The model under review builds one solid part; all positions refer to its coordinate system, in mm. A direction names the side the tool comes from. Give positions to 0.01 mm unless a question says otherwise; leave off trailing zeros. Order: outer loops, then holes, each group sorted by start corner. A loop starts at its lowest first (then second) coordinate and runs counter-clockwise, first axis right, second up.
```python
from build123d import *

# Parameters (mm, degrees)
SKETCH1_R           = 12
SKETCH1_R_2         = 10.5
BOSS_EXTRUDE1_DEPTH = 3
CUT_EXTRUDE1_DEPTH  = 1
CUT_EXTRUDE2_DEPTH  = 3
CUT_EXTRUDE3_DEPTH  = 1


with BuildPart() as part:
    # Sketch1 → Boss-Extrude1 (new body)
    with BuildSketch(Plane(origin=(0, 0, 0), x_dir=(1, 0, 0), z_dir=(0, 1, 0))):
        Circle(SKETCH1_R)
        Circle(SKETCH1_R_2, mode=Mode.SUBTRACT)
    extrude(amount=-BOSS_EXTRUDE1_DEPTH)

    # Sketch6 → Cut-Extrude1 (cut)
    with BuildSketch(Plane(origin=(0, 0, 0), x_dir=(1, 0, 0), z_dir=(0, 1, 0))):
        with BuildLine():
            Line((10.246950766, 4), (11.313708499, 4))
            ThreePointArc((11.313708499, 4), (12, 0), (11.313708499, -4))
            Line((11.313708499, -4), (10.246950766, -4))
            ThreePointArc((10.246950766, -4), (11, 0), (10.246950766, 4))
        make_face()
        with BuildLine():
            Line((-4, 10.246950766), (-4, 11.313708499))
            ThreePointArc((-4, 11.313708499), (0, 12), (4, 11.313708499))
            Line((4, 11.313708499), (4, 10.246950766))
            ThreePointArc((4, 10.246950766), (0, 11), (-4, 10.246950766))
        make_face()
        with BuildLine():
            Line((4, -10.246950766), (4, -11.313708499))
            ThreePointArc((4, -11.313708499), (0, -12), (-4, -11.313708499))
            Line((-4, -11.313708499), (-4, -10.246950766))
            ThreePointArc((-4, -10.246950766), (0, -11), (4, -10.246950766))
        make_face()
        with BuildLine():
            Line((-10.246950766, -4), (-11.313708499, -4))
            ThreePointArc((-11.313708499, -4), (-12, 0), (-11.313708499, 4))
            Line((-11.313708499, 4), (-10.246950766, 4))
            ThreePointArc((-10.246950766, 4), (-11, 0), (-10.246950766, -4))
        make_face()
    extrude(amount=-CUT_EXTRUDE1_DEPTH, mode=Mode.SUBTRACT)

    # Sketch7 → Cut-Extrude2 (cut, through all)
    with BuildSketch(Plane(origin=(0, -1, 0), x_dir=(1, 0, 0), z_dir=(0, 1, 0))):
        with BuildLine():
            Line((-2, 10.816653826), (-2, 11.832159566))
            ThreePointArc((-2, 11.832159566), (0, 12), (2, 11.832159566))
            Line((2, 11.832159566), (2, 10.816653826))
            ThreePointArc((2, 10.816653826), (0, 11), (-2, 10.816653826))
        make_face()
        with BuildLine():
            Line((10.816653826, -2), (11.832159566, -2))
            ThreePointArc((11.832159566, -2), (12, 0), (11.832159566, 2))
            Line((11.832159566, 2), (10.816653826, 2))
            ThreePointArc((10.816653826, 2), (11, 0), (10.816653826, -2))
        make_face()
        with BuildLine():
            Line((-2, -10.816653826), (-2, -11.832159566))
            ThreePointArc((-2, -11.832159566), (0, -12), (2, -11.832159566))
            Line((2, -11.832159566), (2, -10.816653826))
            ThreePointArc((2, -10.816653826), (0, -11), (-2, -10.816653826))
        make_face()
        with BuildLine():
            Line((-10.816653826, 2), (-11.832159566, 2))
            ThreePointArc((-11.832159566, 2), (-12, 0), (-11.832159566, -2))
            Line((-11.832159566, -2), (-10.816653826, -2))
            ThreePointArc((-10.816653826, -2), (-11, 0), (-10.816653826, 2))
        make_face()
    extrude(amount=-CUT_EXTRUDE2_DEPTH, mode=Mode.SUBTRACT)

    # Sketch8 → Cut-Extrude3 (cut)
    with BuildSketch(Plane.XZ.offset(3)):
        with BuildLine():
            Line((-5, -9.233092656), (-5, -10.908712115))
            ThreePointArc((-5, -10.908712115), (-5.764655514, -10.52467324), (-6.5, -10.087120501))
            Line((-6.5, -10.087120501), (-6.5, -8.246211251))
            ThreePointArc((-6.5, -8.246211251), (-5.77113366, -8.771773838), (-5, -9.233092656))
        make_face()
        with BuildLine():
            Line((5, -9.233092656), (5, -10.908712115))
            ThreePointArc((5, -10.908712115), (5.764655514, -10.52467324), (6.5, -10.087120501))
            Line((6.5, -10.087120501), (6.5, -8.246211251))
            ThreePointArc((6.5, -8.246211251), (5.77113366, -8.771773838), (5, -9.233092656))
        make_face()
    extrude(amount=-CUT_EXTRUDE3_DEPTH, mode=Mode.SUBTRACT)


solid = part.part
```
1. Take a section at D-D (x = 3.25). Write out the cut boundary in (y, z).
2. For faces 4 (the flat face through (-4, -0.5, 10.8)), 5 (the flat face through (-6.5, -2.5, -9.2)), 6 (the flat face through (2, -2, 11)), list the 3-axis set-ups (+Z, -Z, +X, -X, +Y, -Y) from which the entire face can be reached by the end or side of a thin tool; tool diameter is ignored.
3. Take a section at C-C (y = -0.55). Write out the cut boundary in (x, z).
4. Insertion check: pin 1 (1.1 mm diameter, centred on y = -0.5, z = -10.5, fed in from +X); pin 2 (0.5 mm diameter, centred on x = 11, z = 3.5, fed in from +Y); pin 3 (0.5 mm diameter, centred on y = -1.5, z = 11, fed in from -X); pin 4 (6 mm diameter, centred on x = -4.5, z = -3, fed in from +Y). Each pin has a flat end and moves straight along its axis. Give the tip position at first contact, or say it passes through.
5. Take a section at B-B (x = 0). Write out the cut boundary in (y, z), and give its area (3 significant figures).
6. To check wall thickness, follow line 1 (Z direction, x = 0, y = -1.7); line 2 (X direction, y = -0.4, z = 6.5). State the ranges of each line that lie inside material, in increasing order.
7. Draft analysis for pull direction X (two halves, no side actions). For faces 1 (the cylindrical face through (-8.41, -1.48, -8.56)), 2 (the flat face through (11, -2, 2)), 3 (the flat face through (4, -0.5, 10.8)), state which applies: pulls with the +X half, pulls with the -X half, needs draft (parallel to the pull), parting line crosses it, or undercut.
8. Take a section at A-A (z = 0). Write out the cut boundary in (x, y), and give its area (3 significant figures).
Answer:
1. outline: (-3, -11.55) - (-1, -11.55) - (-1, -10.51) - (0, -10.51) - (0, -9.98) - (-3, -9.98) - close; (-3, 9.98) - (0, 9.98) - (0, 10.51) - (-1, 10.51) - (-1, 11.55) - (-3, 11.55) - close
2. face 4: +Z, +Y
2. face 5: -Z, -Y
2. face 6: +Z, +Y, -Y
3. outline: (-11.31, -4) arc R12 ccw to (-4, -11.31) - (-4, -10.25) arc R11 ccw to (4, -10.25) - (4, -11.31) arc R12 ccw to (11.31, -4) - (10.25, -4) arc R11 ccw to (10.25, 4) - (11.31, 4) arc R12 ccw to (4, 11.31) - (4, 10.25) arc R11 ccw to (-4, 10.25) - (-4, 11.31) arc R12 ccw to (-11.31, 4) - (-10.25, 4) arc R11 ccw to (-10.25, -4) - close; hole circle Ø21 at (0, 0)
4. pin 1: stops at x = 6.71
4. pin 2: stops at y = -1
4. pin 3: stops at x = -5.33
4. pin 4: passes through
5. outline: (-3, -11) - (0, -11) - (0, -10.5) - (-3, -10.5) - close; (-3, 10.5) - (0, 10.5) - (0, 11) - (-3, 11) - close
5. area: 3.00 mm2
6. line 1: z = -11 to -10.5, 10.5 to 11
6. line 2: x = -10.09 to -8.25, 8.25 to 10.09
7. face 1: pulls with the -X half
7. face 2: needs draft
7. face 3: undercut
8. outline: (-11, -3) - (-10.5, -3) - (-10.5, 0) - (-11, 0) - close; (10.5, -3) - (11, -3) - (11, 0) - (10.5, 0) - close
8. area: 3.00 mm2
